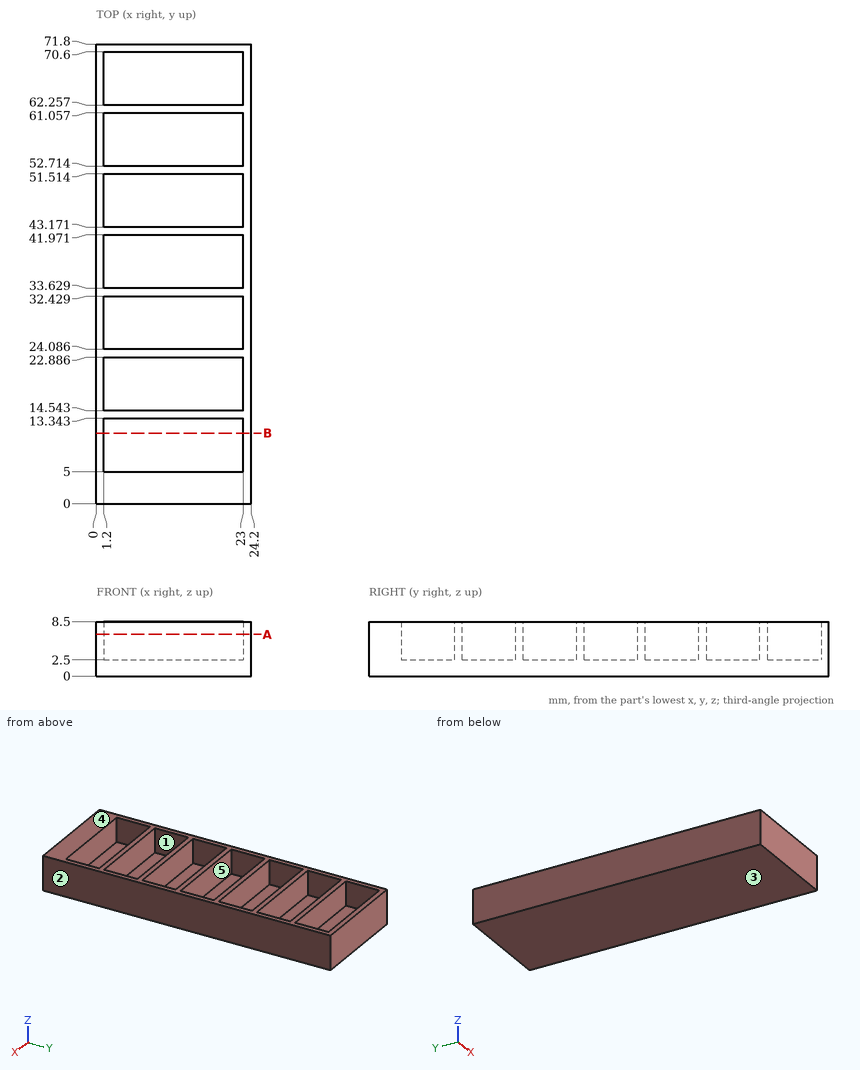
Part print with two shaded views. Sizes in mm from the minimum x, y, z corner. A direction names the side the tool comes from. Round coordinates to 2 decimals unless told otherwise and drop trailing zeros. Order: outer loops, then holes, each group sorted by start corner. A loop starts at its lowest first (then second) coordinate and runs counter-clockwise, first axis right, second up.
(1) Drill centre lines: line 1 (X direction, y = 53, z = 4.5); line 2 (Z direction, x = 15, y = 54). Where is each one in solid material? Low to high.
(2) Band-saw the part on A-A (z = 6.5). Give the number of separate pieces and of enclosed holes in the cut face.
(3) Band-saw the part on B-B (y = 11). List the corners of the cut face in (x, z).
(4) 3-axis set-ups, long thin cutter, end or side, ignore diameter. For the marked faces 4 and 5: which of +Z, -Z, +X, -X, +Y, -Y reach the whole face in a straight line?
(5) Pin check, flat tip, straight feed: pin 1 (4 mm diameter, centred on x = 9.5, y = 9.5, fed in from +Z). Stop position of the tip, or through.
(6) Pull direction X, two halves, no side cores. Call the marked faces 1, 2 and 3: released by +X, released by -X, zero draft, split by the parting line, or undercut.
Verdict:
1. line 1: x = 0 to 1.2, 23 to 24.2
1. line 2: z = 0 to 2.5
2. separate pieces: 1
2. enclosed holes: 7
3. outline: (0, 0) - (24.2, 0) - (24.2, 8.5) - (23, 8.5) - (23, 2.5) - (1.2, 2.5) - (1.2, 8.5) - (0, 8.5) - close
4. face 4: +Z, +X, -X, +Y, -Y
4. face 5: +Z
5. pin 1: stops at z = 2.5
6. face 1: undercut
6. face 2: released by +X
6. face 3: zero draft
